from build123d import *

# Parameters (mm, degrees)
BOX063_W                  = 57
BOX063_H                  = 21
BOX063_DEPTH              = 15
CYLINDER030_R             = 1.75
CYLINDER030_DEPTH         = 24.5
CYLINDER030_PITCH_ANGLE   = 90
CYLINDER031_R             = 3
CYLINDER031_DEPTH         = 21.5
CYLINDER031_PITCH_ANGLE   = 90
FUSION027_PITCH_ANGLE     = -90
FUSION027_PLACEMENT_ANGLE = -180
FUSION024_PITCH_ANGLE     = -90
FUSION024_PLACEMENT_ANGLE = -180
FUSION025_PITCH_ANGLE     = -90
FUSION025_PLACEMENT_ANGLE = -180
BOX029_W                  = 3
BOX029_H                  = 74
BOX029_DEPTH              = 6
BOX029_PITCH_ANGLE        = -90
BOX029_PLACEMENT_ANGLE    = -180
BOX030_W                  = 3
BOX030_H                  = 74
BOX030_DEPTH              = 6
BOX030_PITCH_ANGLE        = -90
BOX030_PLACEMENT_ANGLE    = -180
FUSION026_PITCH_ANGLE     = -90
FUSION026_PLACEMENT_ANGLE = -180
FUSION056_ROLL_ANGLE      = -90
FUSION056_PLACEMENT_ANGLE = 90
CYLINDER_R                = 4
CYLINDER_DEPTH            = 60
CYLINDER063_R             = 1.75
CYLINDER063_DEPTH         = 60
CYLINDER061_R             = 4
CYLINDER061_DEPTH         = 60
CYLINDER060_R             = 4
CYLINDER060_DEPTH         = 60
CYLINDER062_R             = 1.75
CYLINDER062_DEPTH         = 60
SKETCH009_R               = 1.75
PAD007_DEPTH              = 3
PAD008_DEPTH              = 63


with BuildPart() as cube066:
    # Box063 → Box063 (new body)
    with BuildSketch(Plane(origin=(-93, -10.5, -6), x_dir=(1, 0, 0), z_dir=(0, 0, 1))):
        with Locations((28.5, 10.5)):
            Rectangle(BOX063_W, BOX063_H)
    extrude(amount=BOX063_DEPTH)


with BuildPart() as joint_d014:
    # Cylinder030 → Cylinder030 (new body)
    with BuildSketch(Plane.XY):
        Circle(CYLINDER030_R)
    extrude(amount=CYLINDER030_DEPTH)


with BuildPart() as joint_d014_1:
    # Cylinder030 pitch: moved
    add(joint_d014.part.rotate(Axis((0, 0, 0), (0, 1, 0)), CYLINDER030_PITCH_ANGLE))


with BuildPart() as joint_d014_2:
    # Cylinder030 placement: moved
    add(joint_d014_1.part.moved(Location((16, -24.5, 7))))


with BuildPart() as joint_d015:
    # Cylinder031 → Cylinder031 (new body)
    with BuildSketch(Plane.XY):
        Circle(CYLINDER031_R)
    extrude(amount=CYLINDER031_DEPTH)


with BuildPart() as joint_d015_1:
    # Cylinder031 pitch: moved
    add(joint_d015.part.rotate(Axis((0, 0, 0), (0, 1, 0)), CYLINDER031_PITCH_ANGLE))


with BuildPart() as joint_d015_2:
    # Cylinder031 placement: moved
    add(joint_d015_1.part.moved(Location((37, -24.5, 7))))


with BuildPart() as fusion027:
    # Fusion027 base: copy of Joint-D015
    add(joint_d015_2.part)

    # Fusion027: union Joint-D014
    add(joint_d014_2.part)


with BuildPart() as fusion027_1:
    # Fusion027 pitch: moved
    add(fusion027.part.rotate(Axis((0, 0, 0), (0, 1, 0)), FUSION027_PITCH_ANGLE))


with BuildPart() as fusion027_2:
    # Fusion027 placement: moved
    add(fusion027_1.part.moved(Location((-2, -39.5, 0))).rotate(Axis((-2, -39.5, 0), (0, 0, 1)), FUSION027_PLACEMENT_ANGLE))


with BuildPart() as fusion024:
    # Fusion024 base: copy of Joint-D015
    add(joint_d015_2.part)

    # Fusion024: union Joint-D014
    add(joint_d014_2.part)


with BuildPart() as fusion024_1:
    # Fusion024 pitch: moved
    add(fusion024.part.rotate(Axis((0, 0, 0), (0, 1, 0)), FUSION024_PITCH_ANGLE))


with BuildPart() as fusion024_2:
    # Fusion024 placement: moved
    add(fusion024_1.part.moved(Location((-12, 9.5, 0))).rotate(Axis((-12, 9.5, 0), (0, 0, 1)), FUSION024_PLACEMENT_ANGLE))


with BuildPart() as fusion025:
    # Fusion025 base: copy of Joint-D015
    add(joint_d015_2.part)

    # Fusion025: union Joint-D014
    add(joint_d014_2.part)


with BuildPart() as fusion025_1:
    # Fusion025 pitch: moved
    add(fusion025.part.rotate(Axis((0, 0, 0), (0, 1, 0)), FUSION025_PITCH_ANGLE))


with BuildPart() as fusion025_2:
    # Fusion025 placement: moved
    add(fusion025_1.part.moved(Location((-2, 9.5, 0))).rotate(Axis((-2, 9.5, 0), (0, 0, 1)), FUSION025_PLACEMENT_ANGLE))


with BuildPart() as cube047:
    # Box029 → Box029 (new body)
    with BuildSketch(Plane.XY):
        with Locations((1.5, 37)):
            Rectangle(BOX029_W, BOX029_H)
    extrude(amount=BOX029_DEPTH)


with BuildPart() as cube047_1:
    # Box029 pitch: moved
    add(cube047.part.rotate(Axis((0, 0, 0), (0, 1, 0)), BOX029_PITCH_ANGLE))


with BuildPart() as cube047_2:
    # Box029 placement: moved
    add(cube047_1.part.moved(Location((-8, 41.5, 18.5))).rotate(Axis((-8, 41.5, 18.5), (0, 0, 1)), BOX029_PLACEMENT_ANGLE))


with BuildPart() as cube048:
    # Box030 → Box030 (new body)
    with BuildSketch(Plane.XY):
        with Locations((1.5, 37)):
            Rectangle(BOX030_W, BOX030_H)
    extrude(amount=BOX030_DEPTH)


with BuildPart() as cube048_1:
    # Box030 pitch: moved
    add(cube048.part.rotate(Axis((0, 0, 0), (0, 1, 0)), BOX030_PITCH_ANGLE))


with BuildPart() as cube048_2:
    # Box030 placement: moved
    add(cube048_1.part.moved(Location((2, 41.5, 18.5))).rotate(Axis((2, 41.5, 18.5), (0, 0, 1)), BOX030_PLACEMENT_ANGLE))


with BuildPart() as fusion056:
    # Fusion026 base: copy of Joint-D015
    add(joint_d015_2.part)

    # Fusion026: union Joint-D014
    add(joint_d014_2.part)


with BuildPart() as fusion056_1:
    # Fusion026 pitch: moved
    add(fusion056.part.rotate(Axis((0, 0, 0), (0, 1, 0)), FUSION026_PITCH_ANGLE))


with BuildPart() as fusion056_2:
    # Fusion026 placement: moved
    add(fusion056_1.part.moved(Location((-12, -39.5, 0))).rotate(Axis((-12, -39.5, 0), (0, 0, 1)), FUSION026_PLACEMENT_ANGLE))

    # Fusion056: union Fusion027, Fusion024, Fusion025, Cube047, Cube048
    add(fusion027_2.part)
    add(fusion024_2.part)
    add(fusion025_2.part)
    add(cube047_2.part)
    add(cube048_2.part)


with BuildPart() as fusion056_3:
    # Fusion056 roll: moved
    add(fusion056_2.part.rotate(Axis((0, 0, 0), (1, 0, 0)), FUSION056_ROLL_ANGLE))


with BuildPart() as fusion056_4:
    # Fusion056 placement: moved
    add(fusion056_3.part.moved(Location((-30, 0, -2))).rotate(Axis((-30, 0, -2), (0, 0, 1)), FUSION056_PLACEMENT_ANGLE))


with BuildPart() as cylinder:
    # Cylinder → Cylinder (new body)
    with BuildSketch(Plane(origin=(-39, 0, -20), x_dir=(1, 0, 0), z_dir=(0, 0, 1))):
        Circle(CYLINDER_R)
    extrude(amount=CYLINDER_DEPTH)


with BuildPart() as cylinder157:
    # Cylinder063 → Cylinder063 (new body)
    with BuildSketch(Plane(origin=(-8, 0, -12), x_dir=(1, 0, 0), z_dir=(0, 0, 1))):
        Circle(CYLINDER063_R)
    extrude(amount=CYLINDER063_DEPTH)


with BuildPart() as cylinder155:
    # Cylinder061 → Cylinder061 (new body)
    with BuildSketch(Plane(origin=(-8, 0, 4), x_dir=(1, 0, 0), z_dir=(0, 0, 1))):
        Circle(CYLINDER061_R)
    extrude(amount=CYLINDER061_DEPTH)


with BuildPart() as cylinder060:
    # Cylinder060 → Cylinder060 (new body)
    with BuildSketch(Plane(origin=(-20, 0, 4), x_dir=(1, 0, 0), z_dir=(0, 0, 1))):
        Circle(CYLINDER060_R)
    extrude(amount=CYLINDER060_DEPTH)


with BuildPart() as fusion073:
    # Cylinder062 → Cylinder062 (new body)
    with BuildSketch(Plane(origin=(-20, 0, -12), x_dir=(1, 0, 0), z_dir=(0, 0, 1))):
        Circle(CYLINDER062_R)
    extrude(amount=CYLINDER062_DEPTH)

    # Fusion073: union Cylinder157, Cylinder155, Cylinder060
    add(cylinder157.part)
    add(cylinder155.part)
    add(cylinder060.part)


with BuildPart() as pad007:
    # Sketch009 → Pad007 (new body)
    with BuildSketch(Plane.XY.offset(2)):
        with BuildLine():
            Line((-81.932444, 51.697807), (-62, 36))
            Line((-62, 36), (-62, -36))
            Line((-62, -36), (-81.932444, -51.697807))
            ThreePointArc((-81.932444, -51.697807), (-83.267699, -62.932452), (-72.033053, -64.267694))
            Line((-72.033053, -64.267694), (-41.853791, -40.5))
            Line((-41.853791, -40.5), (14, -40.5))
            Line((14, -40.5), (32.837002, -63.104251))
            ThreePointArc((32.837002, -63.104251), (44.104251, -64.12851), (45.12851, -52.861261))
            Line((21, -23.907244), (45.12851, -52.861261))
            Line((21, 23.907244), (21, -23.907244))
            Line((45.12851, 52.861262), (21, 23.907244))
            ThreePointArc((45.12851, 52.861262), (44.104251, 64.12851), (32.837002, 63.104251))
            Line((14, 40.5), (32.837002, 63.104251))
            Line((-41.853791, 40.5), (14, 40.5))
            Line((-72.033053, 64.267694), (-41.853791, 40.5))
            ThreePointArc((-72.033053, 64.267694), (-83.267699, 62.932452), (-81.932444, 51.697807))
        make_face()
        with Locations((-76.982756, 57.982756)):
            Circle(SKETCH009_R, mode=Mode.SUBTRACT)
        with Locations((-76.982756, -57.982756)):
            Circle(SKETCH009_R, mode=Mode.SUBTRACT)
        with Locations((38.982756, 57.982756)):
            Circle(SKETCH009_R, mode=Mode.SUBTRACT)
        with Locations((38.982756, -57.982756)):
            Circle(SKETCH009_R, mode=Mode.SUBTRACT)
    extrude(amount=PAD007_DEPTH)


with BuildPart() as clone_of_cut104:
    # Sketch010 → Pad008 (new body)
    with BuildSketch(Plane(origin=(-62, 2, 0), x_dir=(0, 1, 0), z_dir=(1, 0, 0))):
        Polygon((-35.811086, 2), (-35.811086, 7), (-11, 19.977288), (7, 19.977288), (31.811086, 7), (31.811086, 2), align=None)
    extrude(amount=PAD008_DEPTH)

    # Fusion074: union Pad007
    add(pad007.part)

    # Cut101: cut Fusion073
    add(fusion073.part, mode=Mode.SUBTRACT)

    # Cut102: cut Cylinder
    add(cylinder.part, mode=Mode.SUBTRACT)

    # Cut103: cut Fusion056
    add(fusion056_4.part, mode=Mode.SUBTRACT)

    # Cut104: cut Cube066
    add(cube066.part, mode=Mode.SUBTRACT)


solid = clone_of_cut104.part
For this review, take the finished solid that the model builds, in its own axes (mm). A direction names the side the tool comes from. Coordinates: 2 decimals unless noted, no trailing zeros. Order: outer loops, then holes, each group sorted by start corner. A loop starts at its lowest first (then second) coordinate and runs counter-clockwise, first axis right, second up. Notation, with made-up numbers: (45.25, -29.5) - (81.25, -29.5) arc R23 ccw to (81.25, 1.5) - close; hole circle Ø5 at (50.25, 64). An arc over 180 degrees is marked (long way). Use one line per item in the form item = value.
Q1. Draft analysis for pull direction X (two halves, no side actions). For faces 1 (the flat face through (-7, -2, 4)), 2 (the flat face through (-30.94, 21.23, 13.58)), 3 (the flat face through (21, 0, 3)), 4 (the cylindrical face through (-6.331, 0.526, 2.986)), state which applies: +X half, -X half, draft (parallel to the pull), parting line (faces both ways), or undercut.
Checked values:
face_1 = undercut
face_2 = draft
face_3 = +X half
face_4 = undercut
Q2. For probe 1 along X at (y, z) = (0, 7.5); probe 2 along X at (y, z) = (0, 14.25); probe 3 along X at (y, z) = (0, 3.1), list the stretches that pass through material, from the lowest coordinate up. Write a range as from..to.
Checked values:
probe_1 = -35..-24, -16..-12, -4..1
probe_2 = -62..-43, -35..-24, -16..-12, -4..1
probe_3 = -35..-21.75, -18.25..-9.75, -6.25..21
Q3. Consider section B-B (y = 0). Give the boundary of the cut face in (x, z).
Checked values:
outline = (-62, 9) - (-43, 9) - (-43, 19.98) - (-62, 19.98) - close; (-35, 2) - (-21.75, 2) - (-21.75, 4) - (-24, 4) - (-24, 19.98) - (-35, 19.98) - close; (-18.25, 2) - (-9.75, 2) - (-9.75, 4) - (-12, 4) - (-12, 19.98) - (-16, 19.98) - (-16, 4) - (-18.25, 4) - close; (-6.25, 2) - (21, 2) - (21, 5) - (1, 5) - (1, 19.98) - (-4, 19.98) - (-4, 4) - (-6.25, 4) - close
Q4. Consider section A-A (x = -8). Give the boundary of the cut face in (y, z), then the cut area to 3 significant figures.
Checked values:
outline = (-40.5, 2) - (-1.75, 2) - (-1.75, 4) - (-4, 4) - (-4, 19.98) - (-9, 19.98) - (-33.81, 7) - (-33.81, 5) - (-40.5, 5) - close; (1.75, 2) - (40.5, 2) - (40.5, 5) - (33.81, 5) - (33.81, 7) - (9, 19.98) - (4, 19.98) - (4, 4) - (1.75, 4) - close
area = 799 mm2
Q5. Consider section D-D (y = 17). Give the boundary of the cut face in (x, z), then the cut area to 3 significant figures.
Checked values:
outline = (-62, 2) - (21, 2) - (21, 5) - (1, 5) - (1, 15.79) - (-62, 15.79) - close
area = 929 mm2
Q6. Consider section C-C (x = -28). Give the boundary of the cut face in (y, z), then the cut area to 3 significant figures.
Checked values:
outline = (-40.5, 2) - (40.5, 2) - (40.5, 5) - (33.81, 5) - (33.81, 7) - (9, 19.98) - (-9, 19.98) - (-33.81, 7) - (-33.81, 5) - (-40.5, 5) - close
area = 934 mm2
Q7. For P1, Ø6, axis at x = -35, z = 11.5, coming from the -Y side; P2, Ø2.5, axis at x = -49.5, z = 13.5, coming from the +Y side; P3, Ø5.5, axis at x = -51, z = 6.5, coming from the +Y side, all flat-tipped, find the tip position at first contact; note any pin that passes through.
Checked values:
P1 = -30.94
P2 = 23.77
P3 = 49.52
Q8. For faces 5 (the flat face through (23.287, 51.644, 3.479)), 6 (the flat face through (-49, -10.5, 5)), 7 (the cylindrical face through (-56.68, 6.29, 14.18)), 8 (the flat face through (-50, -8, 15)), 9 (the flat face through (1, 0, 11)), list the 3-axis set-ups (+Z, -Z, +X, -X, +Y, -Y) from which the entire face can be reached by the end or side of a thin tool; tool diameter is ignored.
Checked values:
face_5 = +Z, -Z, +Y
face_6 = -Z, -X
face_7 = -X
face_8 = +Z, -Z
face_9 = +Z, +X, +Y, -Y
